Here's how the part is built. I have some questions about the finished solid (model axes, mm). A direction names the side the tool comes from. Round coordinates to 2 decimals unless told otherwise and drop trailing zeros. Write each loop counter-clockwise with the first axis right and the second up, starting at its lowest first coordinate (ties: lowest second). Pieces come first, ordered by that corner, then holes. Notation, with made-up numbers: (26.5, 19) - (52.5, 19) arc R26 cw to (52.5, 52) - close; hole circle Ø11 at (69.5, 24). An arc over 180 degrees is marked (long way). Use one line per item in the form item = value. Start each with the question number.
1. If I drill on line 1 along X through (y, z) = (2.7, 21); line 2 along X through (y, z) = (1.95, -26.75) (3 decimals); line 3 along Z through (x, y) = (0, 2.2), over which ranges is the centre line in solid material (lowest first)?
2. I want a section at D-D, the plane z = -26.75. List the corners of the cut face in (x, y) for me (1 decimal), plus the area to 3 significant figures.
3. I want a section at A-A, the plane z = 1. List the corners of the cut face in (x, y) for me.
4. Will these pins go through, and if not, where does the flat tip stop? pin 1 (1.3 mm diameter, centred on y = 2.5, z = -6, fed in from +X); pin 2 (2.5 mm diameter, centred on y = 3.5, z = -1.5, fed in from -X); pin 3 (2 mm diameter, centred on y = 2, z = -27.5, fed in from -X); pin 4 (1.5 mm diameter, centred on x = -12.5, z = 19.5, fed in from -Y).
5. Which directions (+Z, -Z, +X, -X, +Y, -Y) give clear straight access to the entire face, cutting with the end or side of a thin tool? Please do faces 4 (the cylindrical face through (43.93, 2.22, -17.87)), 5 (the flat face through (-35, 2, -23.5)), 6 (the conical face through (19.363, 4.635, -23.974)), 7 (the conical face through (-43.756, 4.691, -17.954)).
6. I want a section at B-B, the plane x = -13. List the corners of the cut face in (y, z) for me.
7. We'd pull the mould along X, two halves only. Please class faces 1 (the flat face through (24.8, 2, -28)), 2 (the conical face through (-19.396, 4.635, -24.007)), 3 (the flat face through (-23, 2, 23.5)): +X half, -X half, draft (parallel to the pull), parting line (faces both ways), or undercut.
8. I want a section at C-C, the plane x = 0. List the corners of the cut face in (y, z) for me.
```python
from build123d import *

# Parameters (mm, degrees)
BOSS_EXTRUDE1_DEPTH                                 = 5
CSK_FOR_M2_COUNTERSUNK_FLAT_HEAD_SCREW1_D           = 2.4
CSK_FOR_M2_COUNTERSUNK_FLAT_HEAD_SCREW1_CSINK_D     = 4.4
CSK_FOR_M2_COUNTERSUNK_FLAT_HEAD_SCREW1_CSINK_ANGLE = 90
FILLET2_R                                           = 2
CHAMFER2_SIZE                                       = 0.5
CUT_EXTRUDE1_REACH                                  = 56.314
SKETCH4_W                                           = 70
SKETCH4_H                                           = 30
FILLET3_R                                           = 5


with BuildPart() as part:
    # Sketch1 → Boss-Extrude1 (new body)
    with BuildSketch(Plane(origin=(0, 0, 0), x_dir=(1, 0, 0), z_dir=(0, 1, 0))):
        Polygon((-45, -23.5), (-45, -18.565), (-43.5, -18.565), (-43.5, 18.565), (-45, 18.565), (-45, 23.5), (-24.8, 23.5), (-24.8, 30), (-19.87, 30), (-19.87, 23.5), (19.87, 23.5), (19.87, 30), (24.8, 30), (24.8, 23.5), (45, 23.5), (45, 18.565), (43.5, 18.565), (43.5, -18.565), (45, -18.565), (45, -23.5), (2.465, -23.5), (2.465, -30), (-2.465, -30), (-2.465, -23.5), align=None)
    extrude(amount=BOSS_EXTRUDE1_DEPTH)

    # CSK for M2 Countersunk Flat Head Screw1 (through all)
    with Locations(Plane(origin=(0, 5, 0), x_dir=(1, 0, 0), z_dir=(0, 1, 0))):
        with Locations((0, -26.75), (22.335, 26.75), (-22.335, 26.75), (-42.5, 21), (-42.5, -21), (42.5, 21), (42.5, -21)):
            CounterSinkHole(CSK_FOR_M2_COUNTERSUNK_FLAT_HEAD_SCREW1_D / 2, CSK_FOR_M2_COUNTERSUNK_FLAT_HEAD_SCREW1_CSINK_D / 2, counter_sink_angle=CSK_FOR_M2_COUNTERSUNK_FLAT_HEAD_SCREW1_CSINK_ANGLE)

    # Fillet2
    # the kernel refuses this fillet: 2 mm, written as the material it adds along each edge
    with BuildSketch(Plane(origin=(-2.465, 0, 23.5), x_dir=(0, 0, 1), z_dir=(0, 1, 0))) as fillet2_piece_1:
        with BuildLine():
            CenterArc((FILLET2_R, -FILLET2_R), FILLET2_R, 90, 90)
            Line((0, -FILLET2_R), (0, 0))
            Line((0, 0), (FILLET2_R, 0))
        make_face()
    extrude(amount=5)
    with BuildSketch(Plane(origin=(-43.5, 0, 18.565), x_dir=(0, 0, -1), z_dir=(0, 1, 0)), Plane(origin=(43.5, 0, -18.565), x_dir=(0, 0, 1), z_dir=(0, 1, 0))) as fillet2_piece_2:
        with BuildLine():
            CenterArc((1.936491673, 2), FILLET2_R, 194.477512186, 75.522487814)
            Line((0, 1.5), (0, 0))
            Line((0, 0), (1.936491673, 0))
        make_face()
    extrude(amount=5)
    with BuildSketch(Plane(origin=(-43.5, 0, -18.565), x_dir=(-1, 0, 0), z_dir=(0, 1, 0)), Plane(origin=(43.5, 0, 18.565), x_dir=(1, 0, 0), z_dir=(0, 1, 0))) as fillet2_piece_3:
        with BuildLine():
            CenterArc((2, 1.936491673), FILLET2_R, 180, 75.522487814)
            Line((0, 1.936491673), (0, 0))
            Line((0, 0), (1.5, 0))
        make_face()
    extrude(amount=5)
    with BuildSketch(Plane(origin=(-24.8, 0, -23.5), x_dir=(0, 0, -1), z_dir=(0, 1, 0)), Plane(origin=(-19.87, 0, -23.5), x_dir=(1, 0, 0), z_dir=(0, 1, 0)), Plane(origin=(19.87, 0, -23.5), x_dir=(0, 0, -1), z_dir=(0, 1, 0)), Plane(origin=(24.8, 0, -23.5), x_dir=(1, 0, 0), z_dir=(0, 1, 0)), Plane(origin=(2.465, 0, 23.5), x_dir=(0, 0, 1), z_dir=(0, 1, 0))) as fillet2_piece_4:
        with BuildLine():
            CenterArc((FILLET2_R, FILLET2_R), FILLET2_R, 180, 90)
            Line((0, FILLET2_R), (0, 0))
            Line((0, 0), (FILLET2_R, 0))
        make_face()
    extrude(amount=5)
    # the kernel refuses this fillet: 2 mm, written as the material it takes off along each edge
    with BuildSketch(Plane(origin=(-45, -5, 23.5), x_dir=(0, 0, -1), z_dir=(0, 1, 0)), Plane(origin=(45, -5, -23.5), x_dir=(0, 0, 1), z_dir=(0, 1, 0)), Plane(origin=(45, -5, 23.5), x_dir=(-1, 0, 0), z_dir=(0, 1, 0))) as fillet2_2_piece_1:
        with BuildLine():
            CenterArc((FILLET2_R, -FILLET2_R), FILLET2_R, 90, 90)
            Line((0, -FILLET2_R), (0, 0))
            Line((0, 0), (FILLET2_R, 0))
        make_face()
    extrude(amount=15, mode=Mode.SUBTRACT)
    with BuildSketch(Plane(origin=(-45, -5, -23.5), x_dir=(0, 0, 1), z_dir=(0, 1, 0))) as fillet2_2_piece_2:
        with BuildLine():
            CenterArc((FILLET2_R, FILLET2_R), FILLET2_R, 180, 90)
            Line((0, FILLET2_R), (0, 0))
            Line((0, 0), (FILLET2_R, 0))
        make_face()
    extrude(amount=15, mode=Mode.SUBTRACT)

    # Chamfer2
    # the kernel refuses this chamfer: 0.5 mm, written as the material it takes off along each edge
    with BuildSketch(Plane(origin=(-2.465, 5, 31.285841494), x_dir=(1, 0, 0), z_dir=(0, 0, -1)), Plane(origin=(24.8, 5, -31.285841494), x_dir=(-1, 0, 0), z_dir=(0, 0, 1)), Plane(origin=(-19.87, 5, -31.285841494), x_dir=(-1, 0, 0), z_dir=(0, 0, 1)), Plane(origin=(19.87, 5, -25.5), x_dir=(1, 0, 0), z_dir=(0, 0, -1)), Plane(origin=(2.465, 5, 25.5), x_dir=(-1, 0, 0), z_dir=(0, 0, 1))) as chamfer2_piece_1:
        Polygon((CHAMFER2_SIZE, 0), (0, CHAMFER2_SIZE), (0, 0), align=None)
    extrude(amount=5.785841494, mode=Mode.SUBTRACT)
    with BuildSketch(Plane(origin=(-4.465, 5, 23.5), x_dir=(0, 0, -1), z_dir=(-1, 0, 0)), Plane(origin=(43, 5, 23.5), x_dir=(0, 0, -1), z_dir=(-1, 0, 0))) as chamfer2_piece_2:
        Polygon((CHAMFER2_SIZE, 0), (0, CHAMFER2_SIZE), (0, 0), align=None)
    extrude(amount=38.535, mode=Mode.SUBTRACT)
    with BuildSketch(Plane(origin=(18.584158506, 5, -30), x_dir=(0, 0, 1), z_dir=(1, 0, 0)), Plane(origin=(-26.085841494, 5, -30), x_dir=(0, 0, 1), z_dir=(1, 0, 0)), Plane(origin=(3.750841494, 5, 30), x_dir=(0, 0, -1), z_dir=(-1, 0, 0))) as chamfer2_piece_3:
        Polygon((CHAMFER2_SIZE, 0), (0, CHAMFER2_SIZE), (0, 0), align=None)
    extrude(amount=7.501682988, mode=Mode.SUBTRACT)
    with BuildSketch(Plane(origin=(26.8, 5, -23.5), x_dir=(0, 0, 1), z_dir=(1, 0, 0))) as chamfer2_piece_4:
        Polygon((CHAMFER2_SIZE, 0), (0, CHAMFER2_SIZE), (0, 0), align=None)
    extrude(amount=16.2, mode=Mode.SUBTRACT)
    with BuildSketch(Plane(origin=(-17.87, 5, -23.5), x_dir=(0, 0, 1), z_dir=(1, 0, 0))) as chamfer2_piece_5:
        Polygon((CHAMFER2_SIZE, 0), (0, CHAMFER2_SIZE), (0, 0), align=None)
    extrude(amount=35.74, mode=Mode.SUBTRACT)
    with BuildSketch(Plane(origin=(-43, 5, -23.5), x_dir=(0, -1, 0), z_dir=(1, 0, 0))) as chamfer2_piece_6:
        Polygon((CHAMFER2_SIZE, 0), (0, -CHAMFER2_SIZE), (0, 0), align=None)
    extrude(amount=16.2, mode=Mode.SUBTRACT)
    with BuildSketch(Plane(origin=(-45, 5, -17.279158506), x_dir=(1, 0, 0), z_dir=(0, 0, -1)), Plane(origin=(45, 5, 17.279158506), x_dir=(-1, 0, 0), z_dir=(0, 0, 1)), Plane(origin=(45, 5, -21.5), x_dir=(-1, 0, 0), z_dir=(0, 0, 1)), Plane(origin=(-45, 5, 21.5), x_dir=(1, 0, 0), z_dir=(0, 0, -1))) as chamfer2_piece_7:
        Polygon((CHAMFER2_SIZE, 0), (0, CHAMFER2_SIZE), (0, 0), align=None)
    extrude(amount=4.220841494, mode=Mode.SUBTRACT)
    with BuildSketch(Plane(origin=(-43.5, 5, 16.628508327), x_dir=(1, 0, 0), z_dir=(0, 0, -1)), Plane(origin=(43.5, 5, -16.628508327), x_dir=(-1, 0, 0), z_dir=(0, 0, 1))) as chamfer2_piece_8:
        Polygon((CHAMFER2_SIZE, 0), (0, CHAMFER2_SIZE), (0, 0), align=None)
    extrude(amount=33.257016654, mode=Mode.SUBTRACT)
    with BuildSketch(Plane(origin=(43, 5, 21.5), x_dir=(1, 0, 0), z_dir=(0, 0, -1))) as chamfer2_piece_9:
        Polygon((2 - CHAMFER2_SIZE, 0), (2, CHAMFER2_SIZE), (2, 0), align=None)
    revolve(axis=Axis((43, 5, 21.5), (0, -1, 0)), revolution_arc=90, mode=Mode.SUBTRACT)
    with BuildSketch(Plane(origin=(43, 5, -21.5), x_dir=(0, 0, -1), z_dir=(-1, 0, 0))) as chamfer2_piece_10:
        Polygon((2 - CHAMFER2_SIZE, 0), (2, CHAMFER2_SIZE), (2, 0), align=None)
    revolve(axis=Axis((43, 5, -21.5), (0, -1, 0)), revolution_arc=90, mode=Mode.SUBTRACT)
    with BuildSketch(Plane(origin=(-43, 5, -21.5), x_dir=(-1, 0, 0), z_dir=(0, 0, 1))) as chamfer2_piece_11:
        Polygon((2 - CHAMFER2_SIZE, 0), (2, CHAMFER2_SIZE), (2, 0), align=None)
    revolve(axis=Axis((-43, 5, -21.5), (0, -1, 0)), revolution_arc=90, mode=Mode.SUBTRACT)
    with BuildSketch(Plane(origin=(-43, 5, 21.5), x_dir=(0, 0, 1), z_dir=(1, 0, 0))) as chamfer2_piece_12:
        Polygon((2 - CHAMFER2_SIZE, 0), (2, CHAMFER2_SIZE), (2, 0), align=None)
    revolve(axis=Axis((-43, 5, 21.5), (0, -1, 0)), revolution_arc=90, mode=Mode.SUBTRACT)
    with BuildSketch(Plane(origin=(-4.465, 5, 25.5), x_dir=(1, 0, 0), z_dir=(0, 0, 1))) as chamfer2_piece_13:
        Polygon((2 + CHAMFER2_SIZE, 0), (2, -CHAMFER2_SIZE), (2, 0), align=None)
    revolve(axis=Axis((-4.465, 5, 25.5), (0, 1, 0)), revolution_arc=90, mode=Mode.SUBTRACT)
    with BuildSketch(Plane(origin=(-45.5, 5, 16.628508327), x_dir=(-0.38057900366880315, 0, 0.92474841009134), z_dir=(-0.92474841009134, 0, -0.38057900366880315))) as chamfer2_piece_14:
        Polygon((2 + CHAMFER2_SIZE, 0), (2, -CHAMFER2_SIZE), (2, 0), align=None)
    revolve(axis=Axis((-45.5, 5, 16.628508327), (0, 1, 0)), revolution_arc=112.369552085, mode=Mode.SUBTRACT)
    with BuildSketch(Plane(origin=(-45.5, 5, -16.628508327), x_dir=(1, 0, 0), z_dir=(0, 0, 1))) as chamfer2_piece_15:
        Polygon((2 + CHAMFER2_SIZE, 0), (2, -CHAMFER2_SIZE), (2, 0), align=None)
    revolve(axis=Axis((-45.5, 5, -16.628508327), (0, 1, 0)), revolution_arc=112.369552085, mode=Mode.SUBTRACT)
    with BuildSketch(Plane(origin=(-26.8, 5, -25.5), x_dir=(0, 0, 1), z_dir=(-1, 0, 0))) as chamfer2_piece_16:
        Polygon((2, -CHAMFER2_SIZE), (2 + CHAMFER2_SIZE, 0), (2, 0), align=None)
    revolve(axis=Axis((-26.8, 5, -25.5), (0, 1, 0)), revolution_arc=90, mode=Mode.SUBTRACT)
    with BuildSketch(Plane(origin=(-17.87, 5, -25.5), x_dir=(-1, 0, 0), z_dir=(0, 0, -1))) as chamfer2_piece_17:
        Polygon((2 + CHAMFER2_SIZE, 0), (2, -CHAMFER2_SIZE), (2, 0), align=None)
    revolve(axis=Axis((-17.87, 5, -25.5), (0, 1, 0)), revolution_arc=90, mode=Mode.SUBTRACT)
    with BuildSketch(Plane(origin=(17.87, 5, -25.5), x_dir=(0, 0, 1), z_dir=(-1, 0, 0))) as chamfer2_piece_18:
        Polygon((2 + CHAMFER2_SIZE, 0), (2, -CHAMFER2_SIZE), (2, 0), align=None)
    revolve(axis=Axis((17.87, 5, -25.5), (0, 1, 0)), revolution_arc=90, mode=Mode.SUBTRACT)
    with BuildSketch(Plane(origin=(26.8, 5, -25.5), x_dir=(-1, 0, 0), z_dir=(0, 0, -1))) as chamfer2_piece_19:
        Polygon((2 + CHAMFER2_SIZE, 0), (2, -CHAMFER2_SIZE), (2, 0), align=None)
    revolve(axis=Axis((26.8, 5, -25.5), (0, 1, 0)), revolution_arc=90, mode=Mode.SUBTRACT)
    with BuildSketch(Plane(origin=(45.5, 5, -16.628508327), x_dir=(0.38057900366879954, 0, -0.9247484100913416), z_dir=(0.9247484100913416, 0, 0.38057900366879954))) as chamfer2_piece_20:
        Polygon((2 + CHAMFER2_SIZE, 0), (2, -CHAMFER2_SIZE), (2, 0), align=None)
    revolve(axis=Axis((45.5, 5, -16.628508327), (0, 1, 0)), revolution_arc=112.369552085, mode=Mode.SUBTRACT)
    with BuildSketch(Plane(origin=(45.5, 5, 16.628508327), x_dir=(-1, 0, 0), z_dir=(0, 0, -1))) as chamfer2_piece_21:
        Polygon((2 + CHAMFER2_SIZE, 0), (2, -CHAMFER2_SIZE), (2, 0), align=None)
    revolve(axis=Axis((45.5, 5, 16.628508327), (0, 1, 0)), revolution_arc=112.369552085, mode=Mode.SUBTRACT)
    with BuildSketch(Plane(origin=(4.465, 5, 25.5), x_dir=(0, 0, -1), z_dir=(1, 0, 0))) as chamfer2_piece_22:
        Polygon((2 + CHAMFER2_SIZE, 0), (2, -CHAMFER2_SIZE), (2, 0), align=None)
    revolve(axis=Axis((4.465, 5, 25.5), (0, 1, 0)), revolution_arc=90, mode=Mode.SUBTRACT)
    with BuildSketch(Plane(origin=(-24.8, 5, -25.5), x_dir=(0, -1, 0), z_dir=(0, 0, -1))) as chamfer2_piece_23:
        Polygon((CHAMFER2_SIZE, 0), (0, -CHAMFER2_SIZE), (0, 0), align=None)
    extrude(amount=5.785841494, mode=Mode.SUBTRACT)

    # Sketch4 → Cut-Extrude1 (cut, up to next)
    with BuildSketch(Plane(origin=(0, 5, 0), x_dir=(1, 0, 0), z_dir=(0, 1, 0)), mode=Mode.PRIVATE) as cut_extrude1_sk1:
        Rectangle(SKETCH4_W, SKETCH4_H)
    cut_extrude1_tool1 = extrude(cut_extrude1_sk1.sketch, amount=-CUT_EXTRUDE1_REACH, mode=Mode.PRIVATE) & part.part
    add(cut_extrude1_tool1.solids().sort_by_distance((0, 5, 0))[0], mode=Mode.SUBTRACT)

    # Fillet3
    fillet3_edges = [part.edges().sort_by_distance(p)[0] for p in [
        (35, 2.5, -15),
        (35, 2.5, 15),
        (-35, 2.5, 15),
        (-35, 2.5, -15),
    ]]
    fillet(fillet3_edges, radius=FILLET3_R)


solid = part.part
```
Model answer:
q1.line_1 = -45 to -43.7, -41.3 to 41.3, 43.7 to 45
q1.line_2 = -24.8 to -23.535, -21.135 to -19.87, 19.87 to 21.135, 23.535 to 24.8
q1.line_3 = -23.5 to -15, 15 to 25.55, 27.95 to 30
q2.outline = (-24.8, 0) - (-23.5, 0) - (-23.5, 4) - (-24.4, 4.9) - (-24.8, 4.5) - close; (-21.1, 0) - (-19.9, 0) - (-19.9, 4.5) - (-20.3, 4.9) - (-21.1, 4) - close; (19.9, 0) - (21.1, 0) - (21.1, 4) - (20.3, 4.9) - (19.9, 4.5) - close; (23.5, 0) - (24.8, 0) - (24.8, 4.5) - (24.4, 4.9) - (23.5, 4) - close
q2.area = 22.9 mm2
q3.outline = (-43.5, 0) - (-35, 0) - (-35, 5) - (-43, 5) - (-43.5, 4.5) - close; (35, 0) - (43.5, 0) - (43.5, 4.5) - (43, 5) - (35, 5) - close
q4.pin_1 = 43.5
q4.pin_2 = -43.5
q4.pin_3 = -24.8
q4.pin_4 = 0
q5.face_4 = +X, +Y, -Y
q5.face_5 = -Z, -X, +Y, -Y
q5.face_6 = -Z, +Y
q5.face_7 = -X, +Y
q6.outline = (0, -23.5) - (4.5, -23.5) - (5, -23) - (5, -15) - (0, -15) - close; (0, 15) - (5, 15) - (5, 23) - (4.5, 23.5) - (0, 23.5) - close
q7.face_1 = +X half
q7.face_2 = undercut
q7.face_3 = draft
q8.outline = (0, -23.5) - (4.5, -23.5) - (5, -23) - (5, -15) - (0, -15) - close; (0, 15) - (5, 15) - (5, 24.55) - (4, 25.55) - (0, 25.55) - close; (0, 27.95) - (4, 27.95) - (5, 28.95) - (5, 29.5) - (4.5, 30) - (0, 30) - close
